Could you check a few things on this model? Use its own coordinates, in mm. A direction names the side the tool comes from. Round coordinates to 2 decimals unless told otherwise and drop trailing zeros. Loops run counter-clockwise (first coordinate to the right, second up) from the corner with the lowest first, then second, coordinate; pieces in that order, holes last. Notation, with made-up numbers: (5, 2.5) - (59, 2.5) arc R6 ccw to (59, 13.5) - close; hole circle Ø6 at (-30, 37.25). An arc over 180 degrees is marked (long way). Answer as CSV lines item,"result". Start each with the question number.
1) I'm going to push a flat-ended pin straight in: pin 1 Ø4 at (x, y) = (-4, -5) entering from -Z. Where does the tip first touch, or does it pass through?
2) Suppose I cut it at B-B, the plane y = -20. Write out the boundary of the cut face in (x, z).
3) Suppose I cut it at D-D, the plane z = 0.5. Write out the boundary of the cut face in (x, y).
4) Which directions (+Z, -Z, +X, -X, +Y, -Y) give clear straight access to the entire face, cutting with the end or side of a thin tool? Please do faces 4 (the face through (-0.1, -12.45, 2.5)), 5 (the face through (2.69, -6, 1.48)).
5) Suppose I cut it at A-A, the plane z = 2.55. Write out the boundary of the cut face in (x, y), then the cut area to 3 significant figures.
6) Please list where these lines run through material, in increasing order: line 1 along Y through (x, z) = (4, 1.35); line 2 along X through (y, z) = (4, 1.4); line 3 along X through (y, z) = (-20, 0.75).
7) Suppose I cut it at C-C, the plane x = 0. Write out the boundary of the cut face in (y, z), then the cut area to 3 significant figures.
8) We'd pull the mould along X, two halves only. Please class faces 1 (the face through (-0.215, -18.364, 0.986)), 2 (the face through (0, -1, 3)), 3 (the face through (10, -10, 1)): pulls with the +X half, pulls with the -X half, needs draft (parallel to the pull), parting line crosses it, or undercut.
```python
from build123d import *

# Parameters (mm, degrees)
SKETCH_2_W          = 20
SKETCH_2_H          = 39.5
SKETCH_2_R          = 1.65
EXTRUDE_1_DEPTH     = 3
SKETCH_3_W          = 20
SKETCH_3_H          = 15.1
CUT_EXTRUDE_1_DEPTH = 1
FILLET_2_R          = 5


with BuildPart() as part:
    # ｽｹｯﾁ2 → ﾎﾞｽ - 押し出し1 (new body)
    with BuildSketch(Plane.XY):
        with Locations((0, -9.75)):
            Rectangle(SKETCH_2_W, SKETCH_2_H)
        with Locations((-4, 5)):
            Circle(SKETCH_2_R, mode=Mode.SUBTRACT)
        with Locations((-4, -5)):
            Circle(SKETCH_2_R, mode=Mode.SUBTRACT)
        with Locations((4, -5)):
            Circle(SKETCH_2_R, mode=Mode.SUBTRACT)
        with Locations((4, 5)):
            Circle(SKETCH_2_R, mode=Mode.SUBTRACT)
        with Locations((0, -20)):
            Circle(SKETCH_2_R, mode=Mode.SUBTRACT)
    extrude(amount=EXTRUDE_1_DEPTH)

    # ｽｹｯﾁ3 → ｶｯﾄ - 押し出し1 (cut)
    with BuildSketch(Plane.XY.offset(3)):
        with Locations((0, -20)):
            Rectangle(SKETCH_3_W, SKETCH_3_H)
    extrude(amount=-CUT_EXTRUDE_1_DEPTH, mode=Mode.SUBTRACT)

    # ﾌｨﾚｯﾄ2
    fillet_2_edges = [part.edges().sort_by_distance(p)[0] for p in [
        (-10, -29.5, 1.5),
        (10, -29.5, 1.5),
        (-10, 10, 1.5),
        (10, 10, 1.5),
    ]]
    fillet(fillet_2_edges, radius=FILLET_2_R)


solid = part.part
```
Filled sheet:
1,pin 1,"z = 0"
2,outline,"(-10, 0) - (-1.65, 0) - (-1.65, 2) - (-10, 2) - close; (1.65, 0) - (10, 0) - (10, 2) - (1.65, 2) - close"
3,outline,"(-10, -24.5) arc R5 ccw to (-5, -29.5) - (5, -29.5) arc R5 ccw to (10, -24.5) - (10, 5) arc R5 ccw to (5, 10) - (-5, 10) arc R5 ccw to (-10, 5) - close; hole circle Ø3.3 at (-4, -5); hole circle Ø3.3 at (-4, 5); hole circle Ø3.3 at (0, -20); hole circle Ø3.3 at (4, -5); hole circle Ø3.3 at (4, 5)"
4,face 4,"+Z, +X, -X"
4,face 5,"+Z, -Z"
5,outline,"(-10, -12.45) - (10, -12.45) - (10, 5) arc R5 ccw to (5, 10) - (-5, 10) arc R5 ccw to (-10, 5) - close; (-8.96, -27.55) arc R5 ccw to (-5, -29.5) - (5, -29.5) arc R5 ccw to (8.96, -27.55) - close; hole circle Ø3.3 at (-4, -5); hole circle Ø3.3 at (-4, 5); hole circle Ø3.3 at (4, -5); hole circle Ø3.3 at (4, 5)"
5,area,"434 mm²"
6,line 1,"-29.5 to -6.65, -3.35 to 3.35, 6.65 to 10"
6,line 2,"-10 to -5.31, -2.69 to 2.69, 5.31 to 10"
6,line 3,"-10 to -1.65, 1.65 to 10"
7,outline,"(-29.5, 0) - (-21.65, 0) - (-21.65, 2) - (-27.55, 2) - (-27.55, 3) - (-29.5, 3) - close; (-18.35, 0) - (10, 0) - (10, 3) - (-12.45, 3) - (-12.45, 2) - (-18.35, 2) - close"
7,area,"96.8 mm²"
8,face 1,"undercut"
8,face 2,"needs draft"
8,face 3,"pulls with the +X half"
